Could you check a few things on this drawing? It's one solid part, dimensions in mm from its lowest x, y, z. Round coordinates to 2 decimals unless told otherwise and drop trailing zeros. Write each loop counter-clockwise with the first axis right and the second up, starting at its lowest first coordinate (ties: lowest second). Pieces come first, ordered by that corner, then holes. Notation, with made-up numbers: (61.5, -28.5) -> (105.5, -28.5) arc R16 ccw to (105.5, -19.5) -> close; hole circle Ø8 at (-26.5, 52). An arc over 180 degrees is marked (long way). Answer in a Markdown table with one row per item. Add a question column.
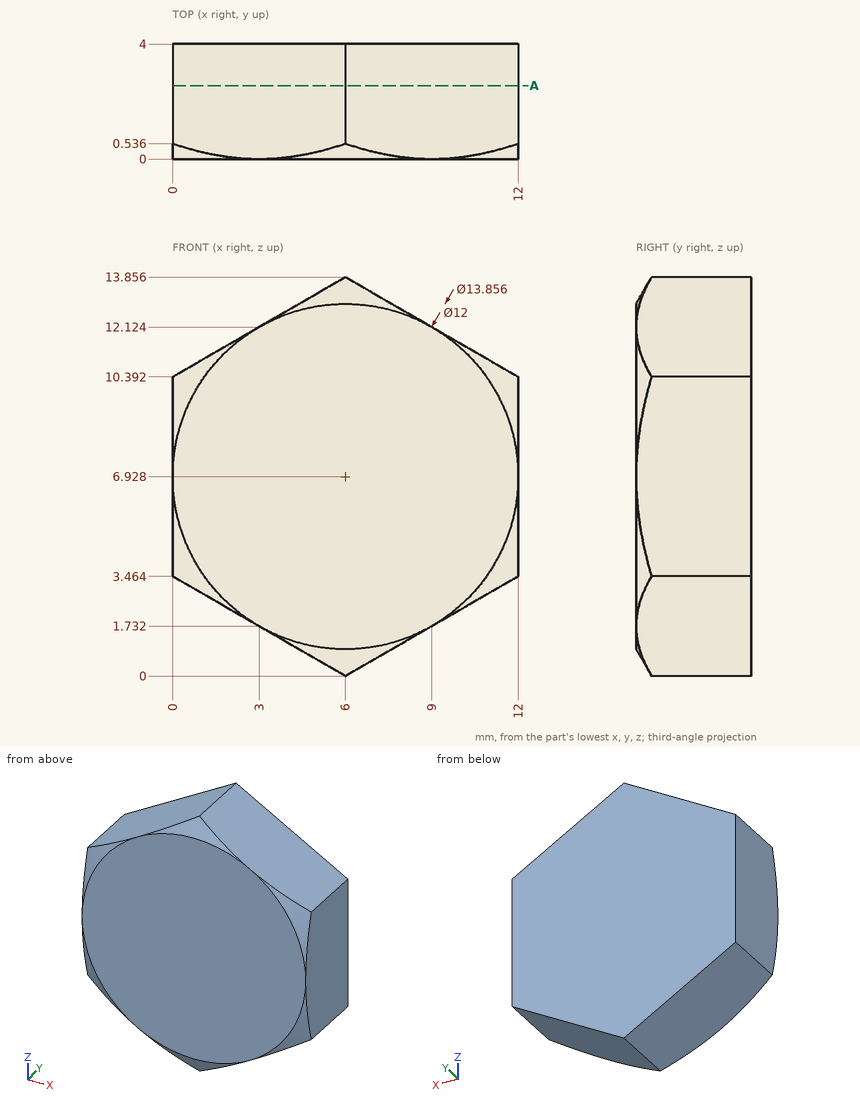
Item 1: If we section it at A-A on y = 2.55: Please give me the cut outline in (x, z).
Item 2: I need wall thicknesses on line 1 along Z through (x, y) = (1, 0.3) (1 decimal); line 2 along X through (y, z) = (3.7, 12.75) (1 decimal); line 3 along Z through (x, y) = (3, 2.2) (1 decimal). Which ranges of each line are inside material? Lowest first, please. Write a range as from..to.
Item 3: For P1, Ø2, axis at x = 1.5, y = 1, coming from the -Z side; P2, Ø1.5, axis at y = 3.5, z = 12, coming from the -X side (1 decimal), each with a flat end and sliding along its axis, tell me the tip position at first contact or that it passes through.
Results list:
| question | item | result |
|---|---|---|
| 1 | outline | (0, 3.46) -> (6, 0) -> (12, 3.46) -> (12, 10.39) -> (6, 13.86) -> (0, 10.39) -> close |
| 2 | line 1 | 2.9..11 |
| 2 | line 2 | 4.1..7.9 |
| 2 | line 3 | 1.7..12.1 |
| 3 | P1 | z = 2.02 |
| 3 | P2 | x = 1.5 |
